Input: dimensioned drawing with shaded views. Units: mm. Origin: part minimum x, y, z. A direction names the side the tool comes from. Give positions to 0.01 mm unless a question says otherwise; leave off trailing zeros. Order: outer loops, then holes, each group sorted by start corner. A loop starts at its lowest first (then second) coordinate and runs counter-clockwise, first axis right, second up. Notation, with made-up numbers: (80, -34) -> (132, -34) arc R8 ccw to (132, -24) -> close; hole circle Ø5 at (-11, 7.25). An arc over 180 degrees is marked (long way). Use CSV: the item, a comma, the result in double quotes.
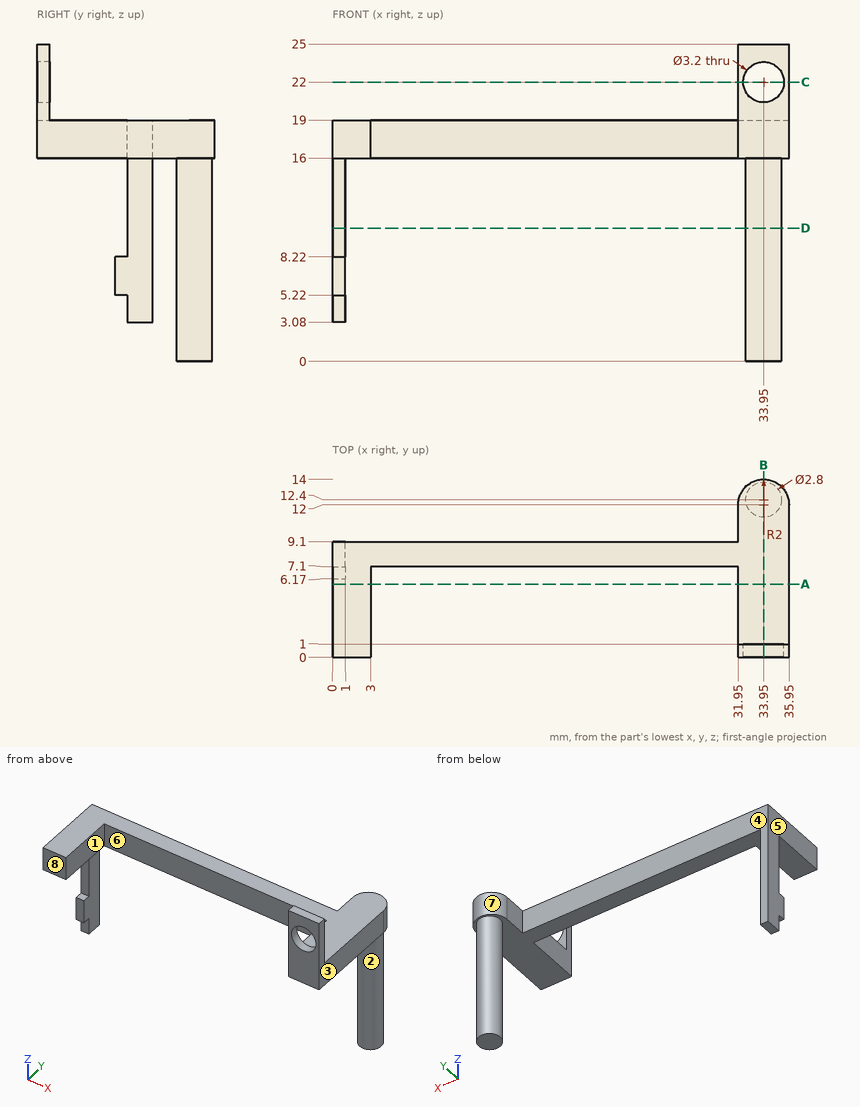
1. Access query for the marked faces 1, 2, 3, 4 and 5. Directions: +Z, -Z, +X, -X, +Y, -Y. A direction counts if a zero-diameter tool reaches every point of the face in a straight line with its end or side. Return the directions, or none.
Answer below:
face 1,"+Z, -Z, -Y"
face 2,"-Z"
face 3,"+Z, -Z, +X, +Y, -Y"
face 4,"+Z, -Z, -X, +Y"
face 5,"+Z, -Z, -X, +Y, -Y"
2. Section query B-B on x = 33.95. Return loops of the section in (y, z), plus the area to 3 significant figures.
Answer below:
outline,"(0, 16) -> (11, 16) -> (11, 0) -> (13.8, 0) -> (13.8, 16) -> (14, 16) -> (14, 19) -> (1, 19) -> (1, 20.4) -> (0, 20.4) -> close; (0, 23.6) -> (1, 23.6) -> (1, 25) -> (0, 25) -> close"
area,"89.6 mm²"
3. Section query C-C on z = 22. Return loops of the section in (x, y).
Answer below:
outline,"(31.95, 0) -> (32.35, 0) -> (32.35, 1) -> (31.95, 1) -> close; (35.55, 0) -> (35.95, 0) -> (35.95, 1) -> (35.55, 1) -> close"
4. Section query D-D on z = 10.5. Return loops of the section in (x, y), plus the area to 3 significant figures.
Answer below:
outline,"(0, 7.1) -> (1, 7.1) -> (1, 9.1) -> (0, 9.1) -> close; circle Ø2.8 at (33.95, 12.4)"
area,"8.16 mm²"
5. Section query A-A on y = 5.75. Return loops of the section in (x, z).
Answer below:
outline,"(0, 16) -> (3, 16) -> (3, 19) -> (0, 19) -> close; (31.95, 16) -> (35.95, 16) -> (35.95, 19) -> (31.95, 19) -> close"
6. Pin query (flat end, axial travel): P1, Ø4, axis at y = 8.5, z = 5.5, coming from the +X side; P2, Ø2, axis at x = 35, z = 21, coming from the +Y side; P3, Ø6, axis at x = 14.5, y = 5.5, coming from the -Z side; P4, Ø1.5, axis at x = 5, y = 6, coming from the +Z side. Return the tip coordinate at first contact, or that it passes through.
Answer below:
P1,"stops at x = 1"
P2,"stops at y = 1"
P3,"stops at z = 16"
P4,"passes through"
7. Ray query, line 1 along Z through (x, y) = (33.95, 0.35); line 2 along X through (y, z) = (0.65, 22); line 3 along Z through (x, y) = (29, 8.25). Return the intervals inside material, ascending.
Answer below:
line 1,"z = 16 to 20.4, 23.6 to 25"
line 2,"x = 31.95 to 32.35, 35.55 to 35.95"
line 3,"z = 16 to 19"
8. Mould query, pull axis X, two halves, no side actions, for the marked faces 6, 7 and 8. Classes: released by +X, released by -X, zero draft, split by the parting line, or undercut.
Answer below:
face 6,"undercut"
face 7,"split by the parting line"
face 8,"zero draft"
